from build123d import *

# Parameters (mm, degrees)
SKETCH1_R           = 0.4
SKETCH1_R_2         = 0.4064
SKETCH1_R_3         = 0.4445
SKETCH1_R_4         = 0.4826
SKETCH1_R_5         = 0.5
SKETCH1_R_6         = 0.508
SKETCH1_R_7         = 0.55
SKETCH1_R_8         = 0.6985
BOSS_EXTRUDE1_DEPTH = 1.5


with BuildPart() as part:
    # Sketch1 → Boss-Extrude1 (new body)
    with BuildSketch(Plane.XY.offset(1.5)):
        with BuildLine():
            Line((190, 33.501164265), (190, 88))
            ThreePointArc((190, 88), (189.414213562, 89.414213562), (188, 90))
            Line((188, 90), (2, 90))
            ThreePointArc((2, 90), (0.585786438, 89.414213562), (0, 88))
            Line((0, 88), (0, 33.501164265))
            ThreePointArc((0, 33.501164265), (0.120614758, 32.817123978), (0.467911114, 32.215589046))
            Line((0.467911114, 32.215589046), (26.90052643, 0.714424781))
            ThreePointArc((26.90052643, 0.714424781), (27.587378793, 0.187384426), (28.432615316, 0))
            Line((28.432615316, 0), (161.567384684, 0))
            ThreePointArc((161.567384684, 0), (162.412621207, 0.187384426), (163.09947357, 0.714424781))
            Line((163.09947357, 0.714424781), (189.532088886, 32.215589046))
            ThreePointArc((189.532088886, 32.215589046), (189.879385242, 32.817123978), (190, 33.501164265))
        make_face()
        with Locations(Location((86.36, 33.655, 0), (0, 0, 180))):
            Circle(SKETCH1_R, mode=Mode.SUBTRACT)
        with Locations(Location((71.12, 33.655, 0), (0, 0, 180))):
            Circle(SKETCH1_R, mode=Mode.SUBTRACT)
        with Locations(Location((76.2, 33.655, 0), (0, 0, 180))):
            Circle(SKETCH1_R, mode=Mode.SUBTRACT)
        with Locations(Location((78.74, 33.655, 0), (0, 0, 180))):
            Circle(SKETCH1_R, mode=Mode.SUBTRACT)
        with Locations(Location((2.54, 47.625, 0), (0, 0, 180))):
            Circle(SKETCH1_R_2, mode=Mode.SUBTRACT)
        with Locations(Location((137.16, 57.785, 0), (0, 0, 180))):
            Circle(SKETCH1_R_2, mode=Mode.SUBTRACT)
        with Locations(Location((142.24, 32.385, 0), (0, 0, 180))):
            Circle(SKETCH1_R_3, mode=Mode.SUBTRACT)
        with Locations(Location((132.08, 42.545, 0), (0, 0, 180))):
            Circle(SKETCH1_R_3, mode=Mode.SUBTRACT)
        with Locations(Location((27.94, 45.085, 0), (0, 0, 180))):
            Circle(SKETCH1_R_3, mode=Mode.SUBTRACT)
        with Locations(Location((27.94, 40.005, 0), (0, 0, 180))):
            Circle(SKETCH1_R_3, mode=Mode.SUBTRACT)
        with Locations(Location((132.08, 40.005, 0), (0, 0, 180))):
            Circle(SKETCH1_R_3, mode=Mode.SUBTRACT)
        with Locations(Location((15.24, 32.385, 0), (0, 0, 180))):
            Circle(SKETCH1_R_3, mode=Mode.SUBTRACT)
        with Locations(Location((102.235, 57.785, 0), (0, 0, 180))):
            Circle(SKETCH1_R_4, mode=Mode.SUBTRACT)
        with Locations(Location((114.935, 47.625, 0), (0, 0, 180))):
            Circle(SKETCH1_R_4, mode=Mode.SUBTRACT)
        with Locations(Location((114.935, 55.245, 0), (0, 0, 180))):
            Circle(SKETCH1_R_4, mode=Mode.SUBTRACT)
        with Locations(Location((117.475, 55.245, 0), (0, 0, 180))):
            Circle(SKETCH1_R_4, mode=Mode.SUBTRACT)
        with Locations(Location((117.475, 50.165, 0), (0, 0, 180))):
            Circle(SKETCH1_R_4, mode=Mode.SUBTRACT)
        with Locations(Location((117.475, 45.085, 0), (0, 0, 180))):
            Circle(SKETCH1_R_4, mode=Mode.SUBTRACT)
        with Locations(Location((117.475, 40.005, 0), (0, 0, 180))):
            Circle(SKETCH1_R_4, mode=Mode.SUBTRACT)
        with Locations(Location((117.475, 34.925, 0), (0, 0, 180))):
            Circle(SKETCH1_R_4, mode=Mode.SUBTRACT)
        with Locations(Location((117.475, 29.845, 0), (0, 0, 180))):
            Circle(SKETCH1_R_4, mode=Mode.SUBTRACT)
        with Locations(Location((117.475, 24.765, 0), (0, 0, 180))):
            Circle(SKETCH1_R_4, mode=Mode.SUBTRACT)
        with Locations(Location((112.395, 24.765, 0), (0, 0, 180))):
            Circle(SKETCH1_R_4, mode=Mode.SUBTRACT)
        with Locations(Location((107.315, 24.765, 0), (0, 0, 180))):
            Circle(SKETCH1_R_4, mode=Mode.SUBTRACT)
        with Locations(Location((102.235, 24.765, 0), (0, 0, 180))):
            Circle(SKETCH1_R_4, mode=Mode.SUBTRACT)
        with Locations(Location((102.235, 29.845, 0), (0, 0, 180))):
            Circle(SKETCH1_R_4, mode=Mode.SUBTRACT)
        with Locations(Location((102.235, 34.925, 0), (0, 0, 180))):
            Circle(SKETCH1_R_4, mode=Mode.SUBTRACT)
        with Locations(Location((102.235, 40.005, 0), (0, 0, 180))):
            Circle(SKETCH1_R_4, mode=Mode.SUBTRACT)
        with Locations(Location((102.235, 45.085, 0), (0, 0, 180))):
            Circle(SKETCH1_R_4, mode=Mode.SUBTRACT)
        with Locations(Location((102.235, 50.165, 0), (0, 0, 180))):
            Circle(SKETCH1_R_4, mode=Mode.SUBTRACT)
        with Locations(Location((43.18, 23.495, 0), (0, 0, 180))):
            Circle(SKETCH1_R_5, mode=Mode.SUBTRACT)
        with Locations(Location((48.26, 23.495, 0), (0, 0, 180))):
            Circle(SKETCH1_R_5, mode=Mode.SUBTRACT)
        with Locations(Location((53.34, 23.495, 0), (0, 0, 180))):
            Circle(SKETCH1_R_5, mode=Mode.SUBTRACT)
        with Locations(Location((120.65, 9.525, 0), (0, 0, 180))):
            Circle(SKETCH1_R_6, mode=Mode.SUBTRACT)
        with Locations(Location((120.65, 6.985, 0), (0, 0, 180))):
            Circle(SKETCH1_R_6, mode=Mode.SUBTRACT)
        with Locations(Location((60.325, 36.195, 0), (0, 0, 180))):
            Circle(SKETCH1_R_6, mode=Mode.SUBTRACT)
        with Locations(Location((60.325, 41.275, 0), (0, 0, 180))):
            Circle(SKETCH1_R_6, mode=Mode.SUBTRACT)
        with Locations(Location((40.64, 12.065, 0), (0, 0, 180))):
            Circle(SKETCH1_R_6, mode=Mode.SUBTRACT)
        with Locations(Location((40.64, 6.985, 0), (0, 0, 180))):
            Circle(SKETCH1_R_6, mode=Mode.SUBTRACT)
        with Locations(Location((5.66, 45.72, 0), (0, 0, 180))):
            Circle(SKETCH1_R_7, mode=Mode.SUBTRACT)
        with Locations(Location((10.16, 39.37, 0), (0, 0, 180))):
            Circle(SKETCH1_R_7, mode=Mode.SUBTRACT)
        with Locations(Location((145.415, 54.665, 0), (0, 0, 180))):
            Circle(SKETCH1_R_7, mode=Mode.SUBTRACT)
        with Locations(Location((139.065, 50.165, 0), (0, 0, 180))):
            Circle(SKETCH1_R_7, mode=Mode.SUBTRACT)
        with Locations(Location((11.1125, 50.165, 0), (0, 0, 180))):
            Circle(SKETCH1_R_8, mode=Mode.SUBTRACT)
        with Locations(Location((24.4475, 34.925, 0), (0, 0, 180))):
            Circle(SKETCH1_R_8, mode=Mode.SUBTRACT)
        with Locations(Location((134.62, 35.8775, 0), (0, 0, 180))):
            Circle(SKETCH1_R_8, mode=Mode.SUBTRACT)
        with Locations(Location((149.86, 49.2125, 0), (0, 0, 180))):
            Circle(SKETCH1_R_8, mode=Mode.SUBTRACT)
        with Locations(Location((134.62, 49.2125, 0), (0, 0, 180))):
            Circle(SKETCH1_R_8, mode=Mode.SUBTRACT)
        with Locations(Location((149.86, 35.8775, 0), (0, 0, 180))):
            Circle(SKETCH1_R_8, mode=Mode.SUBTRACT)
        with Locations(Location((24.4475, 50.165, 0), (0, 0, 180))):
            Circle(SKETCH1_R_8, mode=Mode.SUBTRACT)
        with Locations(Location((11.1125, 34.925, 0), (0, 0, 180))):
            Circle(SKETCH1_R_8, mode=Mode.SUBTRACT)
        with Locations(Location((145.415, 50.165, 0), (0, 0, 180))):
            Circle(SKETCH1_R_7, mode=Mode.SUBTRACT)
        with Locations(Location((139.065, 54.665, 0), (0, 0, 180))):
            Circle(SKETCH1_R_7, mode=Mode.SUBTRACT)
        with Locations(Location((10.16, 45.72, 0), (0, 0, 180))):
            Circle(SKETCH1_R_7, mode=Mode.SUBTRACT)
        with Locations(Location((5.66, 39.37, 0), (0, 0, 180))):
            Circle(SKETCH1_R_7, mode=Mode.SUBTRACT)
        with Locations(Location((120.65, 14.605, 0), (0, 0, 180))):
            Circle(SKETCH1_R_6, mode=Mode.SUBTRACT)
        with Locations(Location((40.64, 9.525, 0), (0, 0, 180))):
            Circle(SKETCH1_R_6, mode=Mode.SUBTRACT)
        with Locations(Location((40.64, 14.605, 0), (0, 0, 180))):
            Circle(SKETCH1_R_6, mode=Mode.SUBTRACT)
        with Locations(Location((60.325, 38.735, 0), (0, 0, 180))):
            Circle(SKETCH1_R_6, mode=Mode.SUBTRACT)
        with Locations(Location((60.325, 33.655, 0), (0, 0, 180))):
            Circle(SKETCH1_R_6, mode=Mode.SUBTRACT)
        with Locations(Location((120.65, 12.065, 0), (0, 0, 180))):
            Circle(SKETCH1_R_6, mode=Mode.SUBTRACT)
        with Locations(Location((40.64, 23.495, 0), (0, 0, 180))):
            Circle(SKETCH1_R_5, mode=Mode.SUBTRACT)
        with Locations(Location((50.8, 23.495, 0), (0, 0, 180))):
            Circle(SKETCH1_R_5, mode=Mode.SUBTRACT)
        with Locations(Location((45.72, 23.495, 0), (0, 0, 180))):
            Circle(SKETCH1_R_5, mode=Mode.SUBTRACT)
        with Locations(Location((102.235, 52.705, 0), (0, 0, 180))):
            Circle(SKETCH1_R_4, mode=Mode.SUBTRACT)
        with Locations(Location((102.235, 47.625, 0), (0, 0, 180))):
            Circle(SKETCH1_R_4, mode=Mode.SUBTRACT)
        with Locations(Location((102.235, 42.545, 0), (0, 0, 180))):
            Circle(SKETCH1_R_4, mode=Mode.SUBTRACT)
        with Locations(Location((102.235, 37.465, 0), (0, 0, 180))):
            Circle(SKETCH1_R_4, mode=Mode.SUBTRACT)
        with Locations(Location((102.235, 32.385, 0), (0, 0, 180))):
            Circle(SKETCH1_R_4, mode=Mode.SUBTRACT)
        with Locations(Location((102.235, 27.305, 0), (0, 0, 180))):
            Circle(SKETCH1_R_4, mode=Mode.SUBTRACT)
        with Locations(Location((104.775, 24.765, 0), (0, 0, 180))):
            Circle(SKETCH1_R_4, mode=Mode.SUBTRACT)
        with Locations(Location((109.855, 24.765, 0), (0, 0, 180))):
            Circle(SKETCH1_R_4, mode=Mode.SUBTRACT)
        with Locations(Location((114.935, 24.765, 0), (0, 0, 180))):
            Circle(SKETCH1_R_4, mode=Mode.SUBTRACT)
        with Locations(Location((117.475, 27.305, 0), (0, 0, 180))):
            Circle(SKETCH1_R_4, mode=Mode.SUBTRACT)
        with Locations(Location((117.475, 32.385, 0), (0, 0, 180))):
            Circle(SKETCH1_R_4, mode=Mode.SUBTRACT)
        with Locations(Location((117.475, 37.465, 0), (0, 0, 180))):
            Circle(SKETCH1_R_4, mode=Mode.SUBTRACT)
        with Locations(Location((117.475, 42.545, 0), (0, 0, 180))):
            Circle(SKETCH1_R_4, mode=Mode.SUBTRACT)
        with Locations(Location((117.475, 47.625, 0), (0, 0, 180))):
            Circle(SKETCH1_R_4, mode=Mode.SUBTRACT)
        with Locations(Location((117.475, 52.705, 0), (0, 0, 180))):
            Circle(SKETCH1_R_4, mode=Mode.SUBTRACT)
        with Locations(Location((117.475, 57.785, 0), (0, 0, 180))):
            Circle(SKETCH1_R_4, mode=Mode.SUBTRACT)
        with Locations(Location((114.935, 50.165, 0), (0, 0, 180))):
            Circle(SKETCH1_R_4, mode=Mode.SUBTRACT)
        with Locations(Location((114.935, 45.085, 0), (0, 0, 180))):
            Circle(SKETCH1_R_4, mode=Mode.SUBTRACT)
        with Locations(Location((102.235, 55.245, 0), (0, 0, 180))):
            Circle(SKETCH1_R_4, mode=Mode.SUBTRACT)
        with Locations(Location((20.32, 32.385, 0), (0, 0, 180))):
            Circle(SKETCH1_R_3, mode=Mode.SUBTRACT)
        with Locations(Location((17.78, 32.385, 0), (0, 0, 180))):
            Circle(SKETCH1_R_3, mode=Mode.SUBTRACT)
        with Locations(Location((27.94, 42.545, 0), (0, 0, 180))):
            Circle(SKETCH1_R_3, mode=Mode.SUBTRACT)
        with Locations(Location((132.08, 45.085, 0), (0, 0, 180))):
            Circle(SKETCH1_R_3, mode=Mode.SUBTRACT)
        with Locations(Location((139.7, 32.385, 0), (0, 0, 180))):
            Circle(SKETCH1_R_3, mode=Mode.SUBTRACT)
        with Locations(Location((144.78, 32.385, 0), (0, 0, 180))):
            Circle(SKETCH1_R_3, mode=Mode.SUBTRACT)
        with Locations(Location((147.32, 57.785, 0), (0, 0, 180))):
            Circle(SKETCH1_R_2, mode=Mode.SUBTRACT)
        with Locations(Location((2.54, 37.465, 0), (0, 0, 180))):
            Circle(SKETCH1_R_2, mode=Mode.SUBTRACT)
        with Locations(Location((81.28, 33.655, 0), (0, 0, 180))):
            Circle(SKETCH1_R, mode=Mode.SUBTRACT)
        with Locations(Location((73.66, 33.655, 0), (0, 0, 180))):
            Circle(SKETCH1_R, mode=Mode.SUBTRACT)
        with Locations(Location((83.82, 33.655, 0), (0, 0, 180))):
            Circle(SKETCH1_R, mode=Mode.SUBTRACT)
        with Locations(Location((88.9, 33.655, 0), (0, 0, 180))):
            Circle(SKETCH1_R, mode=Mode.SUBTRACT)
    extrude(amount=-BOSS_EXTRUDE1_DEPTH)


solid = part.part
Work out the finished part from the listing and answer in its coordinate system (mm). Give positions to 0.01 mm unless a question says otherwise; leave off trailing zeros. Write each loop counter-clockwise with the first axis right and the second up, starting at its lowest first coordinate (ties: lowest second). Pieces come first, ordered by that corner, then holes. Notation, with made-up numbers: (-9.75, -17) - (17.25, -17) arc R24 ccw to (17.25, 8) - close; hole circle Ø8 at (-38, -33.5). An arc over 180 degrees is marked (long way). One line per item, written item: value. Start each with the question number.
1. Find section A-A (z = 0.65). State how many separate pieces and enclosed holes the cut face has, then the cut area to 3 significant figures.
2. Consider probe 1 along Y at (x, z) = (149.86, 0.7); probe 2 along X at (y, z) = (35, 0.7); probe 3 along X at (y, z) = (39.37, 0.4). Determine where each line is inside the solid, lowest interval first.
3. Find section B-B (y = 18). Write down the section's boundary in (x, z).
Geometry results:
1. separate pieces: 1
1. enclosed holes: 95
1. area: 16,100 mm2
2. probe 1: 0 to 35.18, 36.58 to 48.51, 49.91 to 90
2. probe 2: 0 to 10.42, 11.81 to 23.75, 25.14 to 101.76, 102.71 to 117, 117.95 to 190
2. probe 3: 0 to 5.11, 6.21 to 9.61, 10.71 to 190
3. outline: (12.4, 0) - (177.6, 0) - (177.6, 1.5) - (12.4, 1.5) - close
